from build123d import *

# Parameters (mm, degrees)
F1_R     = 8
F1_R_2   = 6.4
F2_DEPTH = 16
F3_DEPTH = 4
F4_DEPTH = 8.7
F6_DEPTH = 1.5


with BuildPart() as f2:
    # F1 (on Top) → F2 (new body)
    with BuildSketch(Plane.XY):
        with Locations((-22, 0)):
            Circle(F1_R)
        with Locations((-22, 0)):
            Circle(F1_R_2, mode=Mode.SUBTRACT)
    extrude(amount=F2_DEPTH)

    # F0 (on Top) → F3 (join)
    with BuildSketch(Plane.XY):
        with BuildLine():
            Line((0, 8), (-22, 8))
            ThreePointArc((-22, 8), (-30, 0), (-22, -8))
            Line((-22, -8), (0, -8))
            Line((0, -8), (0, 8))
        make_face()
    extrude(amount=F3_DEPTH)

    # F4 (add): a face of the model
    f4_faces = [f2.faces().sort_by_distance(p)[0] for p in [
        (-22, 0, 4),
    ]]
    extrude(f4_faces, amount=F4_DEPTH)

    # F5 (on Front) → F6 (join, symmetric)
    with BuildSketch(Plane.XZ):
        Polygon((-8.2692483334, 4), (-14.318941161, 10.031673433), (-14.3099449018, 4), align=None)
    extrude(amount=F6_DEPTH, both=True)

    # F7: F2 across plane


with BuildPart() as f2_1:
    add(f2.part)
    add(f2.part.mirror(Plane.YZ))


solid = f2_1.part
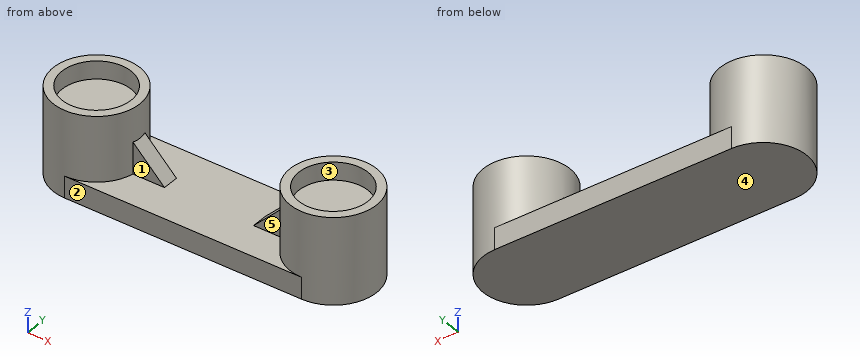
Here's how the part is built. I have some questions about the finished solid (model axes, mm). Face numbers are marked on the shaded views. A direction names the side the tool comes from. Give positions to 0.01 mm unless a question says otherwise; leave off trailing zeros. Order: outer loops, then holes, each group sorted by start corner. A loop starts at its lowest first (then second) coordinate and runs counter-clockwise, first axis right, second up. Notation, with made-up numbers: M 53.5,-12 L 58.5,-12 A20 cw 58.5,9 Z; hole C 4.5,10.5 d5. An arc over 180 degrees is marked long. Answer as a JSON object with one key per item and string values. Group by question number.
1) Suppose I cut it at C-C, the plane y = 0. Write out the boundary of the cut face in (x, z).
2) Suppose I cut it at D-D, the plane x = 24. Write out the boundary of the cut face in (y, z).
3) On a 3-axis mill with a long thin cutter (end or side, diameter ignored), from which of +Z, -Z, +X, -X, +Y, -Y can I reach the whole of each face in a straight line? I mean the marked faces 1, 2 and 3. Say none if no direction works.
4) Suppose I cut it at B-B, the plane x = -19.5. Write out the boundary of the cut face in (y, z).
5) We'd pull the mould along X, two halves only. Please class the marked faces 4 and 5: pulls with the +X half, pulls with the -X half, needs draft (parallel to the pull), parting line crosses it, or undercut.
6) I'm going to push flat-ended pins straight in: pin 1 Ø3 at (y, z) = (-0.5, 2) entering from -X; pin 2 Ø1.8 at (x, z) = (-12, 5.5) entering from +Y; pin 3 Ø4 at (x, y) = (8, 4.5) entering from +Z; pin 4 Ø4.5 at (x, z) = (-11, 6.5) entering from -Y. Where does each tip first touch, or does it pass through?
7) Suppose I cut it at A-A, the plane z = 14. Write out the boundary of the cut face in (x, y), plus the area to 3 significant figures.
8) Please list where these lines run through material, in increasing order: L1, parallel to X at y = 0, z = 14.8; L2, parallel to Y at x = -22, z = 14.6; L3, parallel to X at y = 4, z = 14.75. Write a range as [from, to].
Results found:
{
 "1": {"outline": "M -30,0 L 30,0 L 30,16 L 28.4,16 L 28.4,12.7 L 15.6,12.7 L 15.6,16 L 14,16 L 14,9.71 L 8.27,4 L -8.27,4 L -14,9.71 L -14,16 L -15.6,16 L -15.6,12.7 L -28.4,12.7 L -28.4,16 L -30,16 Z"},
 "2": {"outline": "M -7.75,0 L 7.75,0 L 7.75,16 L 6.08,16 L 6.08,12.7 L -6.08,12.7 L -6.08,16 L -7.75,16 Z"},
 "3": {"face 1": "+Z, -Y", "face 2": "+Z, -Z, +X, -X, -Y", "face 3": "+Z"},
 "4": {"outline": "M -8,0 L 8,0 L 8,4 L 7.6,4 L 7.6,16 L 5.89,16 L 5.89,12.7 L -5.89,12.7 L -5.89,16 L -7.6,16 L -7.6,4 L -8,4 Z"},
 "5": {"face 4": "needs draft", "face 5": "undercut"},
 "6": {"pin 1": "x = -30", "pin 2": "y = 1.5", "pin 3": "z = 4", "pin 4": "y = -1.5"},
 "7": {"outline": "C -22,0 d16; C 22,0 d16; hole C -22,0 d12.8; hole C 22,0 d12.8", "area": "145 mm²"},
 "8": {"L1": "[-30, -28.4], [-15.6, -14], [14, 15.6], [28.4, 30]", "L2": "[-8, -6.4], [6.4, 8]", "L3": "[-28.93, -27], [-17, -15.07], [15.07, 17], [27, 28.93]"}
}
